from build123d import *

# Parameters (mm, degrees)
CUT_EXTRUDE3_DEPTH      = 37.462309307
CUT_EXTRUDE3_DEPTH_BACK = 37.462309307
SKETCH2_R               = 2
CUT_EXTRUDE4_DEPTH      = 37.462309307
FILLET1_R               = 4
FILLET2_R               = 5


with BuildPart() as part:
    # Sketch1 → Revolve1 (revolve)
    with BuildSketch(Plane.XY, mode=Mode.PRIVATE) as revolve1_sk:
        with BuildLine():
            Line((-5.196152423, 12), (-8.196152423, 12))
            Line((-8.196152423, 12), (-8.196152423, 10))
            Line((-8.196152423, 10), (-10.196152423, 10))
            Line((-10.196152423, 10), (-10.196152423, 0.8))
            Line((-10.196152423, 0.8), (-23.5, 0.8))
            Line((-23.5, 0.8), (-23.5, 0))
            Line((-23.5, 0), (0, 0))
            Line((0, 0), (0, 15))
            ThreePointArc((0, 15), (-3, 14.196152423), (-5.196152423, 12))
        make_face()
    revolve(revolve1_sk.sketch.rotate(Axis((0, 0, 0), (0, 1, 0)), 270), axis=Axis((0, 0, 0), (0, 1, 0)))

    # Sketch2 → Cut-Extrude3 (cut, two sides: drawn at the far end of the back side and taken through both)
    with BuildSketch(Plane(origin=(0, 0, 0), x_dir=(1, 0, 0), z_dir=(0, 1, 0)).offset(-CUT_EXTRUDE3_DEPTH_BACK)):
        with Locations(Location((-17.5, 0, 0), (0, 0, 270))):
            Circle(SKETCH2_R)
        with Locations(Location((17.5, 0, 0), (0, 0, 270))):
            Circle(SKETCH2_R)
    extrude(amount=CUT_EXTRUDE3_DEPTH + CUT_EXTRUDE3_DEPTH_BACK, mode=Mode.SUBTRACT)

    # Sketch3 → Cut-Extrude4 (cut, through all)
    with BuildSketch(Plane(origin=(0, 0, 0), x_dir=(1, 0, 0), z_dir=(0, 1, 0))):
        with BuildLine():
            Line((-23.307724042, 3), (0, 12))
            Line((0, 12), (23.307724042, 3))
            ThreePointArc((23.307724042, 3), (0, 23.5), (-23.307724042, 3))
        make_face()
        with BuildLine():
            Line((0, -12), (23.307724042, -3))
            ThreePointArc((23.307724042, -3), (0, -23.5), (-23.307724042, -3))
            Line((-23.307724042, -3), (0, -12))
        make_face()
    extrude(amount=CUT_EXTRUDE4_DEPTH, mode=Mode.SUBTRACT)

    # Fillet1
    fillet1_edges = [part.edges().sort_by_distance(p)[0] for p in [
        (23.307724042, 0.4, -3),
        (-23.307724042, 0.4, -3),
        (-23.307724042, 0.4, 3),
        (23.307724042, 0.4, 3),
    ]]
    fillet(fillet1_edges, radius=FILLET1_R)

    # Fillet2
    fillet2_edges = [part.edges().sort_by_distance(p)[0] for p in [
        (0, 0.4, -12),
        (0, 0.4, 12),
    ]]
    fillet(fillet2_edges, radius=FILLET2_R)


solid = part.part
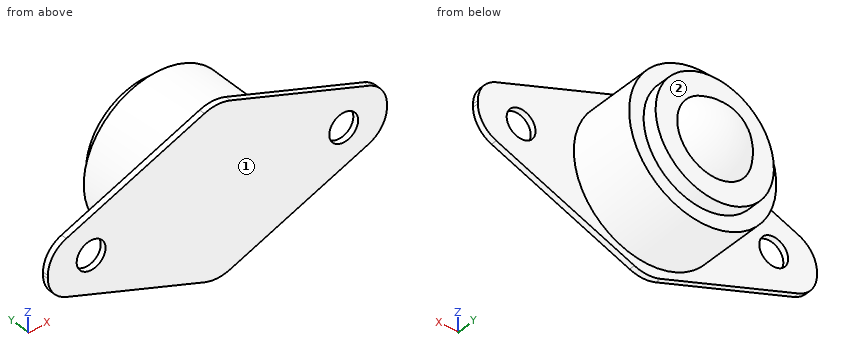
Source: CAD feature listing. Evaluate the final solid. Frame: model axes, mm. Face numbers are marked on the shaded views. A direction names the side the tool comes from. Round coordinates to 2 decimals unless told otherwise and drop trailing zeros. Write each loop counter-clockwise with the first axis right and the second up, starting at its lowest first coordinate (ties: lowest second). Pieces come first, ordered by that corner, then holes. Notation, with made-up numbers: M 47,36 L 79,36 A25 cw 79,63 Z; hole C 68.5,33.25 d7. An arc over 180 degrees is marked long. One line per item, written item: value. Start each with the question number.
Item 1: Section query A-A (z = -1). Return the cut outline in (x, y), plus the area to 3 significant figures.
Item 2: Section query D-D (y = 9). Return the cut outline in (x, z), plus the area to 3 significant figures.
Item 3: Section query B-B (x = -17.5). Return the cut outline in (y, z), plus the area to 3 significant figures.
Item 4: Set-up query: the marked faces 1 and 2. Return all of +Z, -Z, +X, -X, +Y, -Y with unobstructed straight access to the full face (end or side cutting, diameter ignored); none if empty.
Item 5: Section query C-C (x = 0). Return the cut outline in (y, z), plus the area to 3 significant figures.
Item 6: Ray query, L1, parallel to X at y = 0.5, z = 0; L2, parallel to Y at x = -16.5, z = 2.5; L3, parallel to Z at x = -17.5, y = 0.5. Return the intervals inside material, ascending. Write a range as from..to.
Item 7: Pin query (flat end, axial travel): pin 1 (6 mm diameter, centred on y = 8.5, z = 5.5, fed in from -X); pin 2 (1 mm diameter, centred on y = 8.5, z = -2, fed in from -X); pin 3 (2 mm diameter, centred on x = 17.5, y = 1.5, fed in from -Z); pin 4 (2.5 mm diameter, centred on x = -17.5, z = 0, fed in from -Y). Return the tip coordinate at first contact, or that it passes through.
Result set:
1. outline: M -23.41,0 L -19.23,0 L -19.23,0.8 L -23.41,0.8 Z; M -15.77,0 L 15.77,0 L 15.77,0.8 L 10.15,0.8 L 10.15,10 L 8.13,10 L 8.13,12 L 5.1,12 A5.92 ccw -5.1,12 L -8.13,12 L -8.13,10 L -10.15,10 L -10.15,0.8 L -15.77,0.8 Z; M 19.23,0 L 23.41,0 L 23.41,0.8 L 19.23,0.8 Z
1. area: 272 mm²
2. outline: C 0,0 d20.39
2. area: 327 mm²
3. outline: M 0,-5.24 L 0.8,-5.24 L 0.8,-2 L 0,-2 Z; M 0,2 L 0.8,2 L 0.8,5.24 L 0,5.24 Z
3. area: 5.19 mm²
4. face 1: +Z, -Z, +X, -X, -Y
4. face 2: +Y
5. outline: M 0,-11.64 L 0.8,-11.64 L 0.8,-10.2 L 10,-10.2 L 10,-8.2 L 12,-8.2 L 12,-5.2 A6 ccw 12,5.2 L 12,8.2 L 10,8.2 L 10,10.2 L 0.8,10.2 L 0.8,11.64 L 0,11.64 Z
5. area: 261 mm²
6. L1: x = -23.5..-19.5, -15.5..15.5, 19.5..23.5
6. L2: y = 0..0.8
6. L3: z = -5.24..-2, 2..5.24
7. pin 1: stops at x = -9.88
7. pin 2: stops at x = -10.09
7. pin 3: stops at z = -5.52
7. pin 4: passes through
